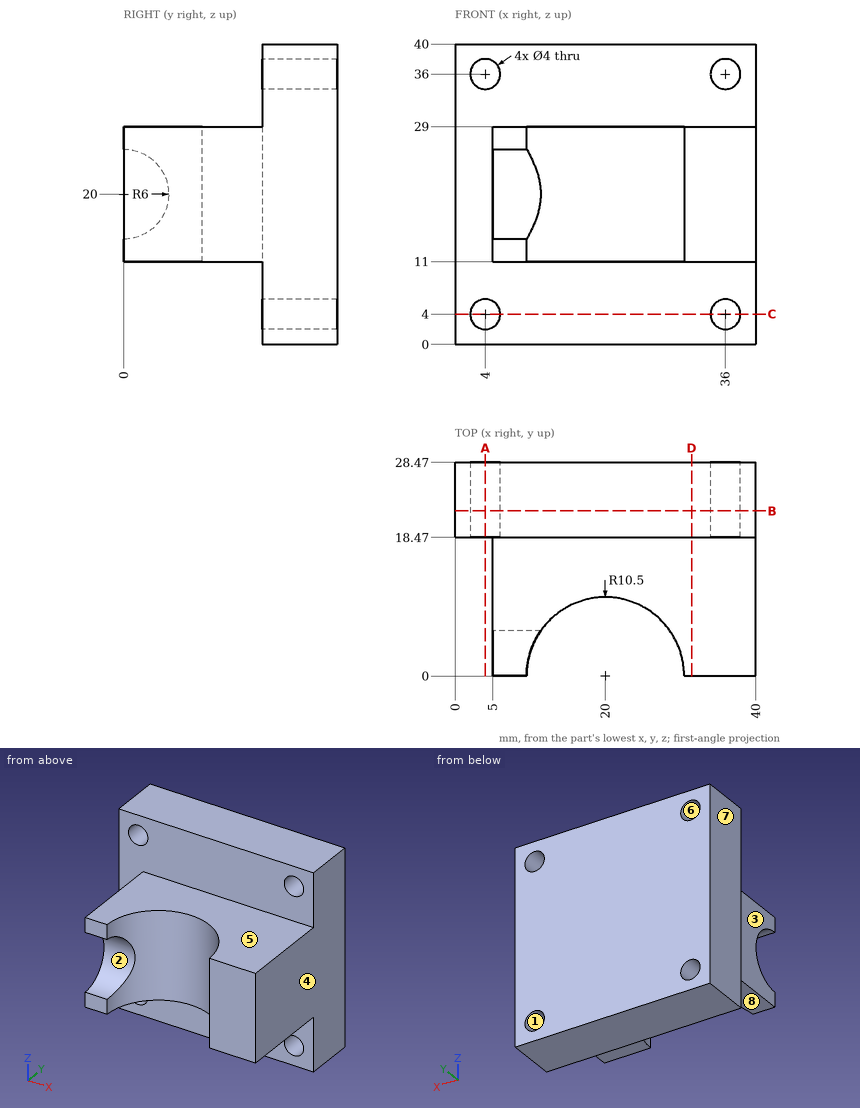
The drawing under review shows one solid part. Ordinate dimensions are in mm from its lowest x, y, z. A direction names the side the tool comes from. Round coordinates to 2 decimals unless told otherwise and drop trailing zeros. Write each loop counter-clockwise with the first axis right and the second up, starting at its lowest first coordinate (ties: lowest second). Pieces come first, ordered by that corner, then holes. Notation, with made-up numbers: M -30.75,15 L -16.75,15 A13 ccw -16.75,32 Z; hole C 34.5,86 d2. An arc over 180 degrees is marked long. One line per item, written item: value. Start each with the question number.
(1) Wall thickness on line 1 (Z direction, x = 36, y = 22.75); line 2 (X direction, y = 21, z = 35); line 3 (X direction, y = 7.75, z = 15.5): over which ranges is each line inside the solid? List them lowest first.
(2) We need section A-A (x = 4). Give the boundary of the cut face in (y, z), and give its area (3 significant figures).
(3) Insertion check: pin 1 (2.5 mm diameter, centred on x = 36, z = 36, fed in from -Y); pin 2 (5 mm diameter, centred on x = 7.5, y = 3, fed in from -Z); pin 3 (6.5 mm diameter, centred on x = 4, z = 36, fed in from -Y); pin 4 (1 mm diameter, centred on y = 14.5, z = 25, fed in from -X). Each pin has a flat end and moves straight along its axis. Give the tip position at first contact, or say it passes through.
(4) The part is to be moulded in two halves that separate along X. For the marked faces 6, 7 and 8, say which applies: released by +X, released by -X, zero draft, split by the parting line, or undercut.
(5) We need section D-D (x = 31.5). Give the boundary of the cut face in (y, z).
(6) We need section C-C (z = 4). Give the boundary of the cut face in (x, y).
(7) We need section B-B (y = 22). Give the boundary of the cut face in (x, z).
(8) Machinability: for the marked faces 1, 2, 3, 4 and 5, which of the approach directions +Z, -Z, +X, -X, +Y, -Y give a long, thin tool a straight path to every point of the face, cutting with its end or side? Answer none if there is none.
Result:
1. line 1: 0 to 2, 6 to 34, 38 to 40
1. line 2: 0 to 2.27, 5.73 to 34.27, 37.73 to 40
1. line 3: 5 to 12.92, 27.08 to 40
2. outline: M 18.47,0 L 28.47,0 L 28.47,2 L 18.47,2 Z; M 18.47,6 L 28.47,6 L 28.47,34 L 18.47,34 Z; M 18.47,38 L 28.47,38 L 28.47,40 L 18.47,40 Z
2. area: 320 mm²
3. pin 1: through
3. pin 2: z = 11
3. pin 3: y = 18.47
3. pin 4: x = 5
4. face 6: undercut
4. face 7: released by -X
4. face 8: zero draft
5. outline: M 0,11 L 18.47,11 L 18.47,0 L 28.47,0 L 28.47,40 L 18.47,40 L 18.47,29 L 0,29 Z
6. outline: M 0,18.47 L 2,18.47 L 2,28.47 L 0,28.47 Z; M 6,18.47 L 34,18.47 L 34,28.47 L 6,28.47 Z; M 38,18.47 L 40,18.47 L 40,28.47 L 38,28.47 Z
7. outline: M 0,0 L 40,0 L 40,40 L 0,40 Z; hole C 4,4 d4; hole C 4,36 d4; hole C 36,4 d4; hole C 36,36 d4
8. face 1: +Y, -Y
8. face 2: -X, -Y
8. face 3: +Z, -Z, -X, -Y
8. face 4: +Z, -Z, +X, +Y, -Y
8. face 5: +Z, +X, -X, -Y
